Geometry: final body of the model. Coordinates: model frame, mm. Face numbers are marked on the shaded views. A direction names the side the tool comes from. Give positions to 0.01 mm unless a question says otherwise; leave off trailing zeros. Loops run counter-clockwise (first coordinate to the right, second up) from the corner with the lowest first, then second, coordinate; pieces in that order, holes last. Notation, with made-up numbers: (26.25, 15.5) -> (35.25, 15.5) arc R22 ccw to (35.25, 39.5) -> close; hole circle Ø11 at (30, 47). An arc over 180 degrees is marked (long way). One line per question, with ' | ' between items. Start each with the question number.
Item 1: Material intervals for line 1 along X through (y, z) = (1.55, 0); line 2 along Y through (x, z) = (8, 17.9); line 3 along Z through (x, y) = (5.5, -1), sorted ascending. Write a range as [from, to].
Item 2: Pin query (flat end, axial travel): P1, Ø8, axis at x = 6, z = 6.5, coming from the -Y side; P2, Ø5, axis at x = -8, y = -7, coming from the +Z side; P3, Ø2.5, axis at x = 8, y = -7, coming from the -Z side. Return the tip coordinate at first contact, or that it passes through.
Item 3: Section B-B on x = 0. Return loops of the section in (y, z).
Item 4: Section C-C on x = -9.5. Return loops of the section in (y, z).
Item 5: Mould query, pull axis Y, two halves, no side actions, for the marked faces 1, 2, 3 and 4. Classes: released by +Y, released by -Y, zero draft, split by the parting line, or undercut.
Item 6: Section D-D on y = -14. Return loops of the section in (x, z), then the cut area to 3 significant figures.
Item 7: Section A-A on y = -7. Return loops of the section in (x, z).
Item 8: Set-up query: the marked faces 5 and 6. Return all of +Z, -Z, +X, -X, +Y, -Y with unobstructed straight access to the full face (end or side cutting, diameter ignored); none if empty.
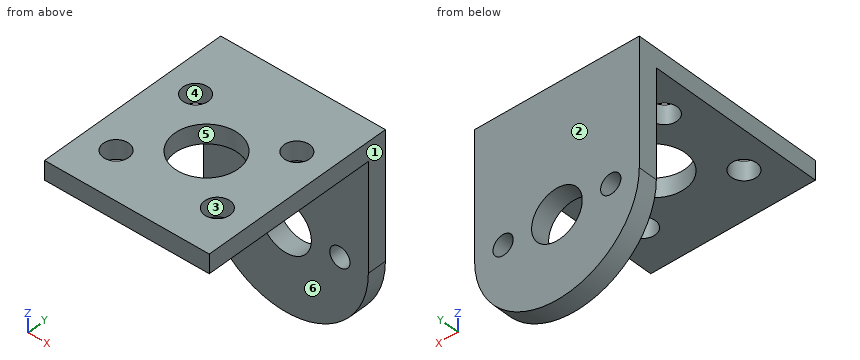
from build123d import *

# Parameters (mm, degrees)
SKETCH_1_R      = 4
SKETCH_1_R_2    = 1.6
EXTRUDE_1_DEPTH = 3
SKETCH_3_W      = 26
SKETCH_3_H      = 31
SKETCH_3_R      = 5
SKETCH_3_R_2    = 2
EXTRUDE_2_DEPTH = 3


with BuildPart() as part:
    # 草图1 → 凸台-拉伸1 (new body)
    with BuildSketch(Plane(origin=(0, 0, 0), x_dir=(1, 0, 0), z_dir=(0, 1, 0))):
        with BuildLine():
            Line((-13, 0), (-13, -20))
            Line((-13, -20), (13, -20))
            Line((13, -20), (13, 0))
            ThreePointArc((13, 0), (0, 13), (-13, 0))
        make_face()
        with Locations(Location((0, 0, 0), (0, 0, 270))):
            Circle(SKETCH_1_R, mode=Mode.SUBTRACT)
        with Locations(Location((-8.5, 0, 0), (0, 0, 270))):
            Circle(SKETCH_1_R_2, mode=Mode.SUBTRACT)
        with Locations(Location((8.5, 0, 0), (0, 0, 270))):
            Circle(SKETCH_1_R_2, mode=Mode.SUBTRACT)
    extrude(amount=EXTRUDE_1_DEPTH)

    # 草图3 → 凸台-拉伸2 (add)
    with BuildSketch(Plane.XY.offset(20)):
        with Locations((0, -12.5)):
            Rectangle(SKETCH_3_W, SKETCH_3_H)
        with Locations((0, -14)):
            Circle(SKETCH_3_R, mode=Mode.SUBTRACT)
        with Locations((-8, -7)):
            Circle(SKETCH_3_R_2, mode=Mode.SUBTRACT)
        with Locations((8, -7)):
            Circle(SKETCH_3_R_2, mode=Mode.SUBTRACT)
        with Locations((8, -21)):
            Circle(SKETCH_3_R_2, mode=Mode.SUBTRACT)
        with Locations((-8, -21)):
            Circle(SKETCH_3_R_2, mode=Mode.SUBTRACT)
    extrude(amount=-EXTRUDE_2_DEPTH)


solid = part.part
Result sheet:
1) line 1: x = [-13, -10.1], [-6.9, -4], [4, 6.9], [10.1, 13] | line 2: y = [-28, -23], [-19, -9], [-5, 3] | line 3: z = [17, 20]
2) P1: stops at y = 0 | P2: stops at z = 20 | P3: passes through
3) outline: (-28, 17) -> (-19, 17) -> (-19, 20) -> (-28, 20) -> close; (-9, 17) -> (0, 17) -> (0, 4) -> (3, 4) -> (3, 20) -> (-9, 20) -> close; (0, -13) -> (3, -13) -> (3, -4) -> (0, -4) -> close
4) outline: (-28, 17) -> (-22.32, 17) -> (-22.32, 20) -> (-28, 20) -> close; (-19.68, 17) -> (-8.32, 17) -> (-8.32, 20) -> (-19.68, 20) -> close; (-5.68, 17) -> (0, 17) -> (0, 1.25) -> (3, 1.25) -> (3, 20) -> (-5.68, 20) -> close; (0, -8.87) -> (3, -8.87) -> (3, -1.25) -> (0, -1.25) -> close
5) face 1: zero draft | face 2: released by +Y | face 3: undercut | face 4: undercut
6) outline: (-13, 17) -> (-5, 17) -> (-5, 20) -> (-13, 20) -> close; (5, 17) -> (13, 17) -> (13, 20) -> (5, 20) -> close | area: 48.0 mm²
7) outline: (-13, 17) -> (-10, 17) -> (-10, 20) -> (-13, 20) -> close; (-6, 17) -> (6, 17) -> (6, 20) -> (-6, 20) -> close; (10, 17) -> (13, 17) -> (13, 20) -> (10, 20) -> close
8) face 5: +Z, -Z | face 6: -Z, +X, -X, -Y
